Can you work these out from the model? Positions are in its coordinate system, mm. A direction names the side the tool comes from. Give positions to 0.01 mm unless a question says otherwise; leave off trailing zeros. Order: outer loops, then holes, each group sorted by start corner. A loop starts at its lowest first (then second) coordinate and runs counter-clockwise, first axis right, second up. Notation, with made-up numbers: (54, -7.75) - (80, -7.75) arc R34 cw to (80, 31.25) - close; hole circle Ø8 at (-10, 47). An arc over 180 degrees is marked (long way). Use one line per item in the form item = value. Start each with the question number.
1) Please list where these lines run through material, in increasing order: probe 1 along X at (y, z) = (85, 21); probe 2 along X at (y, z) = (149.5, 17.5); probe 3 along Z at (x, y) = (53, 123.5).
2) We'd pull the mould along X, two halves only. Please class faces 6 (the flat face through (165, 112, 10)), 7 (the flat face through (10.487, 111, 35)), 8 (the flat face through (113, 0, 5)): released by +X, released by -X, zero draft, split by the parting line, or undercut.
3) Suppose I cut it at C-C, the plane z = 47. Write out the boundary of the cut face in (x, y), and give its area (3 significant figures).
4) Suppose I cut it at A-A, the plane y = 111. Write out the boundary of the cut face in (x, z), and give its area (3 significant figures).
5) For pin 1 (11 mm diameter, centred on x = 51.5, y = 13.5, fed in from +Z); pin 2 (3 mm diameter, centred on x = 27, z = 21.5, fed in from +Y); pin 3 (2 mm diameter, centred on x = 53.5, y = 194, fed in from +Z), each with a flat end and sliding along its axis, tell me the tip position at first contact or that it passes through.
6) Suppose I cut it at D-D, the plane y = 191. Write out the boundary of the cut face in (x, z).
7) Suppose I cut it at B-B, the plane x = 91.5. Write out the boundary of the cut face in (y, z), and give its area (3 significant figures).
8) Which directions (+Z, -Z, +X, -X, +Y, -Y) give clear straight access to the entire face, cutting with the end or side of a thin tool? Please do faces 1 (the flat face through (86.487, 106, 35)), 2 (the flat face through (195, 72.5, 17)), 3 (the flat face through (195, 147.5, 17)), 4 (the flat face through (53, 10, 24)), 5 (the flat face through (53, 15, 25)).
```python
from build123d import *

# Parameters (mm, degrees)
ESQUISSE1_W        = 230
ESQUISSE1_H        = 220
BOSS_EXTRU_1_DEPTH = 10
BOSS_EXTRU_2_DEPTH = 50
ESQUISSE3_W        = 66
ESQUISSE3_H        = 10
BOSS_EXTRU_3_DEPTH = 15
ESQUISSE4_W        = 50
ESQUISSE4_H        = 75
ESQUISSE4_W_2      = 30
ESQUISSE4_H_2      = 55
BOSS_EXTRU_4_DEPTH = 15


with BuildPart() as part:
    # Esquisse1 → Boss.-Extru.1 (new body)
    with BuildSketch(Plane.XY):
        with Locations((115, 110)):
            Rectangle(ESQUISSE1_W, ESQUISSE1_H)
    extrude(amount=BOSS_EXTRU_1_DEPTH)

    # Esquisse2 → Boss.-Extru.2 (add)
    with BuildSketch(Plane.XY.offset(10)):
        Polygon((10.487156365, 10), (20.487156365, 10), (20.487156365, 200), (86.487156365, 200), (86.487156365, 10), (96.487156365, 10), (96.487156365, 210), (86.487156365, 210), (20.487156365, 210), (10.487156365, 210), align=None)
    extrude(amount=BOSS_EXTRU_2_DEPTH)

    # Esquisse3 → Boss.-Extru.3 (add)
    with BuildSketch(Plane.XY.offset(10)):
        with Locations((53.487156365, 15)):
            Rectangle(ESQUISSE3_W, ESQUISSE3_H)
    extrude(amount=BOSS_EXTRU_3_DEPTH)

    # Esquisse4 → Boss.-Extru.4 (add)
    with BuildSketch(Plane.XY.offset(10)):
        with Locations((195, 110)):
            Rectangle(ESQUISSE4_W, ESQUISSE4_H)
        with Locations((195, 110)):
            Rectangle(ESQUISSE4_W_2, ESQUISSE4_H_2, mode=Mode.SUBTRACT)
    extrude(amount=BOSS_EXTRU_4_DEPTH)


solid = part.part
```
Result sheet:
q1.probe_1 = 10.49 to 20.49, 86.49 to 96.49, 170 to 180, 210 to 220
q1.probe_2 = 10.49 to 20.49, 86.49 to 96.49
q1.probe_3 = 0 to 10
q2.face_6 = undercut
q2.face_7 = released by -X
q2.face_8 = zero draft
q3.outline = (10.49, 10) - (20.49, 10) - (20.49, 200) - (86.49, 200) - (86.49, 10) - (96.49, 10) - (96.49, 210) - (10.49, 210) - close
q3.area = 4,660 mm²
q4.outline = (0, 0) - (230, 0) - (230, 10) - (220, 10) - (220, 25) - (210, 25) - (210, 10) - (180, 10) - (180, 25) - (170, 25) - (170, 10) - (96.49, 10) - (96.49, 60) - (86.49, 60) - (86.49, 10) - (20.49, 10) - (20.49, 60) - (10.49, 60) - (10.49, 10) - (0, 10) - close
q4.area = 3,600 mm²
q5.pin_1 = 25
q5.pin_2 = 210
q5.pin_3 = 10
q6.outline = (0, 0) - (230, 0) - (230, 10) - (96.49, 10) - (96.49, 60) - (86.49, 60) - (86.49, 10) - (20.49, 10) - (20.49, 60) - (10.49, 60) - (10.49, 10) - (0, 10) - close
q7.outline = (0, 0) - (220, 0) - (220, 10) - (210, 10) - (210, 60) - (10, 60) - (10, 10) - (0, 10) - close
q7.area = 12,200 mm²
q8.face_1 = +Z
q8.face_2 = +Z, +X, -Y
q8.face_3 = +Z, +X, +Y
q8.face_4 = +Z, +X, -X, -Y
q8.face_5 = +Z, -Y
